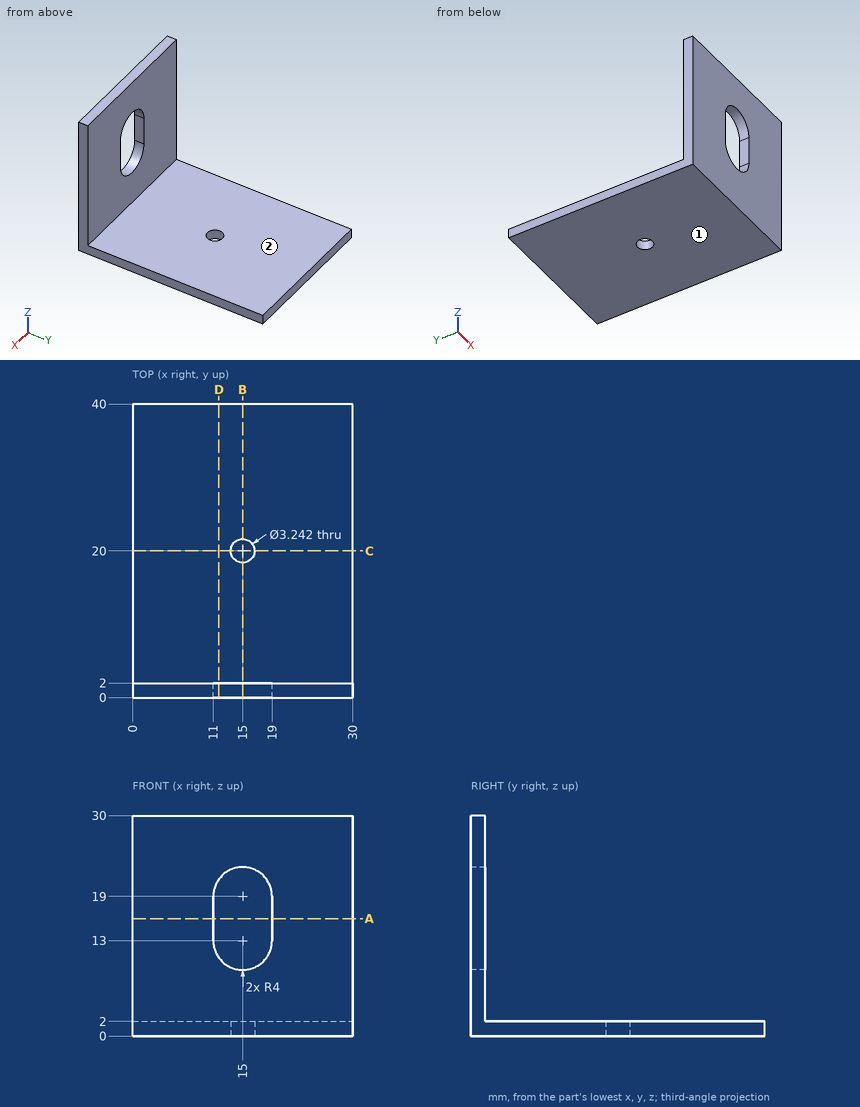
Geometry check sheet. Reference: drawing and pictorial views, mm from the part's lowest x, y, z. A direction names the side the tool comes from. Round coordinates to 2 decimals unless told otherwise and drop trailing zeros. Write each loop counter-clockwise with the first axis right and the second up, starting at its lowest first coordinate (ties: lowest second). Pieces come first, ordered by that corner, then holes. Notation, with made-up numbers: (27, 13) -> (36, 13) arc R14 cw to (36, 36) -> close; hole circle Ø11 at (41.5, 5.5). An arc over 180 degrees is marked (long way). Put each result on its own line as item: value.
1) Thickness scan on probe 1 along X at (y, z) = (20, 1.3); probe 2 along Y at (x, z) = (15, 0.5); probe 3 along Z at (x, y) = (5.5, 4). Record the ranges inside material, lowest first. Write a range as from..to.
Recorded:
probe 1: x = 0..13.38, 16.62..30
probe 2: y = 0..18.38, 21.62..40
probe 3: z = 0..2
2) Cross-section at D-D, the plane x = 11.75. Enter the section's corners in (y, z).
Recorded:
outline: (0, 0) -> (40, 0) -> (40, 2) -> (2, 2) -> (2, 10.67) -> (0, 10.67) -> close; (0, 21.33) -> (2, 21.33) -> (2, 30) -> (0, 30) -> close
3) Cross-section at A-A, the plane z = 16. Enter the section's corners in (x, y).
Recorded:
outline: (0, 0) -> (11, 0) -> (11, 2) -> (0, 2) -> close; (19, 0) -> (30, 0) -> (30, 2) -> (19, 2) -> close
4) Cross-section at C-C, the plane y = 20. Enter the section's corners in (x, z).
Recorded:
outline: (0, 0) -> (13.38, 0) -> (13.38, 2) -> (0, 2) -> close; (16.62, 0) -> (30, 0) -> (30, 2) -> (16.62, 2) -> close
5) Depth check by flat-ended pin: P1, Ø0.6, axis at y = 1.5, z = 16, coming from the -X side; P2, Ø5, axis at x = 23.5, y = 31.5, coming from the +Z side; P3, Ø8.5, axis at x = 20.5, z = 9, coming from the +Y side; P4, Ø8, axis at y = 13.5, z = 7.5, coming from the +X side. Enter the tip coordinate at first touch or a pass-through.
Recorded:
P1: stops at x = 0
P2: stops at z = 2
P3: stops at y = 2
P4: passes through
6) Cross-section at B-B, the plane x = 15. Enter the section's corners in (y, z).
Recorded:
outline: (0, 0) -> (18.38, 0) -> (18.38, 2) -> (2, 2) -> (2, 9) -> (0, 9) -> close; (0, 23) -> (2, 23) -> (2, 30) -> (0, 30) -> close; (21.62, 0) -> (40, 0) -> (40, 2) -> (21.62, 2) -> close
7) Access from +Z, -Z, +X, -X, +Y, -Y to the whole of each face (thin tool, end or side, straight path). Record for the marked faces 1 and 2.
Recorded:
face 1: -Z, +X, -X, +Y, -Y
face 2: +Z, +X, -X, +Y
